For this review, take the finished solid that the model builds, in its own axes (mm). A direction names the side the tool comes from. Round coordinates to 2 decimals unless told otherwise and drop trailing zeros. Write each loop counter-clockwise with the first axis right and the second up, starting at its lowest first coordinate (ties: lowest second). Pieces come first, ordered by that corner, then holes.
from build123d import *

# Parameters (mm, degrees)
CROQUIS3_W               = 75.27
CROQUIS3_H               = 32.91
SALIENTE_EXTRUIR1_DEPTH  = 3.82
SALIENTE_EXTRUIR2_DEPTH  = 3.84
SALIENTE_EXTRUIR3_DEPTH  = 3.84
CROQUIS8_W               = 82.95
CROQUIS8_H               = 15.57
SALIENTE_EXTRUIR5_DEPTH  = 3.8
CROQUIS9_W               = 82.95
CROQUIS9_H               = 24.43
SALIENTE_EXTRUIR7_DEPTH  = 3.8
CROQUIS10_W              = 82.95
CROQUIS10_H              = 8.18
SALIENTE_EXTRUIR9_DEPTH  = 33.8
CROQUIS11_R              = 3.475
CORTAR_EXTRUIR3_DEPTH    = 33.8
SALIENTE_EXTRUIR10_DEPTH = 3.84
SALIENTE_EXTRUIR11_DEPTH = 3.84
CROQUIS15_R              = 3.9
SALIENTE_EXTRUIR12_DEPTH = 3.8


with BuildPart() as part:
    # Croquis3 → Saliente-Extruir1 (new body)
    with BuildSketch(Plane.XY):
        Rectangle(CROQUIS3_W, CROQUIS3_H)
    extrude(amount=SALIENTE_EXTRUIR1_DEPTH)

    # Croquis4 → Saliente-Extruir2 (add)
    with BuildSketch(Plane(origin=(37.635, 0, 0), x_dir=(0, 0, -1), z_dir=(1, 0, 0))):
        Polygon((-3.82, -16.455), (0, -16.455), (0, 16.455), (-3.82, 16.455), (-15.57, -16.455), align=None)
    extrude(amount=SALIENTE_EXTRUIR2_DEPTH)

    # Croquis5 → Saliente-Extruir3 (add)
    with BuildSketch(Plane.ZY.offset(37.635)):
        Polygon((3.82, -16.455), (0, -16.455), (0, 16.455), (3.82, 16.455), (15.57, -16.455), align=None)
    extrude(amount=SALIENTE_EXTRUIR3_DEPTH)

    # Croquis8 → Saliente-Extruir5 (add)
    with BuildSketch(Plane(origin=(0, -16.455, 0), x_dir=(-1, 0, 0), z_dir=(0, -1, 0))):
        with Locations((0, -7.785)):
            Rectangle(CROQUIS8_W, CROQUIS8_H)
    extrude(amount=SALIENTE_EXTRUIR5_DEPTH)

    # Croquis9 → Saliente-Extruir7 (add)
    with BuildSketch(Plane.XZ.offset(20.255)):
        with Locations((0, -12.215)):
            Rectangle(CROQUIS9_W, CROQUIS9_H)
    extrude(amount=-SALIENTE_EXTRUIR7_DEPTH)

    # Croquis10 → Saliente-Extruir9 (add)
    with BuildSketch(Plane(origin=(0, 16.455, 0), x_dir=(1, 0, 0), z_dir=(0, 1, 0))):
        with Locations((0, 4.09)):
            Rectangle(CROQUIS10_W, CROQUIS10_H)
    extrude(amount=-SALIENTE_EXTRUIR9_DEPTH)

    # Croquis11 → Cortar-Extruir3 (cut)
    with BuildSketch(Plane.XY.offset(3.82)):
        Circle(CROQUIS11_R)
    extrude(amount=-CORTAR_EXTRUIR3_DEPTH, mode=Mode.SUBTRACT)

    # Croquis12 → Saliente-Extruir10 (add)
    with BuildSketch(Plane(origin=(41.475, 0, 0), x_dir=(0, 0, -1), z_dir=(1, 0, 0))):
        Polygon((8.18, 16.455), (24.43, -16.455), (8.18, -16.455), align=None)
    extrude(amount=-SALIENTE_EXTRUIR10_DEPTH)

    # Croquis14 → Saliente-Extruir11 (add)
    with BuildSketch(Plane.ZY.offset(41.475)):
        Polygon((-8.18, 16.455), (-8.18, -16.772028127), (-24.43, -16.455), align=None)
    extrude(amount=-SALIENTE_EXTRUIR11_DEPTH)

    # Croquis15 → Saliente-Extruir12 (add)
    # profile 1 of 2: a face of its own
    with BuildSketch(Plane.XZ.offset(20.255)):
        with BuildLine():
            Line((41.475, 15.57), (41.475, -24.43))
            Line((41.475, -24.43), (52.99576157, -14.32670597))
            Line((52.99576157, -14.32670597), (52.99576157, -14.522664239))
            ThreePointArc((52.99576157, -14.522664239), (63.088425809, -4.43), (52.99576157, 5.662664239))
            Line((52.99576157, 5.662664239), (52.99576157, 5.858622508))
            Line((52.99576157, 5.858622508), (41.475, 15.57))
        make_face()
        with Locations(Location((52.99576157, -4.43, 0), (0, 0, 270))):
            Circle(CROQUIS15_R, mode=Mode.SUBTRACT)
    # profile 2 of 2: a face of its own
    with BuildSketch(Plane.XZ.offset(20.255)):
        with BuildLine():
            Line((-52.99576157, 5.858622508), (-41.475, 15.57))
            Line((-41.475, 15.57), (-41.475, -24.43))
            Line((-41.475, -24.43), (-52.99576157, -14.32670597))
            Line((-52.99576157, -14.32670597), (-52.99576157, -14.522664239))
            ThreePointArc((-52.99576157, -14.522664239), (-63.088425809, -4.43), (-52.99576157, 5.662664239))
            Line((-52.99576157, 5.662664239), (-52.99576157, 5.858622508))
        make_face()
        with Locations(Location((-52.99576157, -4.43, 0), (0, 0, 270))):
            Circle(CROQUIS15_R, mode=Mode.SUBTRACT)
    extrude(amount=-SALIENTE_EXTRUIR12_DEPTH)


solid = part.part
(1) For line 1 along X through (y, z) = (-18, -4); line 2 along Y through (x, z) = (0, -1.5) (3 decimals); line 3 along X through (y, z) = (0.5, -8.5) (3 decimals), list the stretches that pass through material, from the lowest coordinate up.
Geometry check:
line 1: x = -63.08 to -56.87, -49.12 to 49.12, 56.87 to 63.08
line 2: y = -20.255 to -3.475, 3.475 to 16.455
line 3: x = -41.475 to -37.635, 37.635 to 41.475
(2) We need section D-D, the plane x = 39. Give the boundary of the cut face in (y, z) (3 decimals).
Geometry check:
outline: (-20.255, -24.43) - (-16.455, -24.43) - (16.455, -8.18) - (16.455, 3.82) - (-16.455, 15.57) - (-20.255, 15.57) - close
(3) We need section B-B, the plane x = 0. Give the boundary of the cut face in (y, z) (3 decimals).
Geometry check:
outline: (-20.255, -24.43) - (-16.455, -24.43) - (-16.455, -8.18) - (-3.475, -8.18) - (-3.475, 3.82) - (-16.455, 3.82) - (-16.455, 15.57) - (-20.255, 15.57) - close; (3.475, -8.18) - (16.455, -8.18) - (16.455, 3.82) - (3.475, 3.82) - close
(4) For pin 1 Ø10 at (x, y) = (14, -5.5) entering from -Z; pin 2 Ø24 at (x, z) = (-57.5, -6) entering from +Y (3 decimals); pin 3 Ø6 at (y, z) = (9.5, 8) entering from +X (3 decimals); pin 4 Ø7 at (x, z) = (53, -4.43) entering from -Y, all flat-tipped, find the tip position at first contact; note any pin that passes through.
Geometry check:
pin 1: stops at z = -8.18
pin 2: stops at y = -16.455
pin 3: stops at x = 41.475
pin 4: passes through
(5) Mouldability with a two-part tool opening along X and no side actions: class faces 4 (the face through (-1, -18, -24.43)), 5 (the face through (41.475, -3, -5)), 6 (the face through (-63.086, -18.382, -4.652)), 7 (the face through (-1, 4, -8.18)) as pulls with the +X half, pulls with the -X half, needs draft (parallel to the pull), parting line crosses it, or undercut.
Geometry check:
face 4: needs draft
face 5: pulls with the +X half
face 6: pulls with the -X half
face 7: undercut
(6) We need section C-C, the plane y = 0. Give the boundary of the cut face in (x, z) (3 decimals), and give its area (3 significant figures).
Geometry check:
outline: (-41.475, -16.305) - (-37.635, -16.305) - (-37.635, -8.18) - (-3.475, -8.18) - (-3.475, 3.82) - (-37.635, 3.82) - (-37.635, 9.695) - (-41.475, 9.695) - close; (3.475, -8.18) - (37.635, -8.18) - (37.635, -16.305) - (41.475, -16.305) - (41.475, 9.695) - (37.635, 9.695) - (37.635, 3.82) - (3.475, 3.82) - close
area: 1,020 mm2
(7) We need section A-A, the plane z = -4.43. Give the boundary of the cut face in (x, y) (3 decimals).
Geometry check:
outline: (-63.088, -20.255) - (-56.896, -20.255) - (-56.896, -16.455) - (-63.088, -16.455) - close; (-49.096, -20.255) - (49.096, -20.255) - (49.096, -16.455) - (41.475, -16.455) - (41.475, 16.455) - (-41.475, 16.455) - (-41.475, -16.455) - (-49.096, -16.455) - close; (56.896, -20.255) - (63.088, -20.255) - (63.088, -16.455) - (56.896, -16.455) - close; hole circle Ø6.95 at (0, 0)
(8) For faces 1 (the face through (-1, -16.455, -16)), 2 (the face through (-39.58, -0.23, -16.42)), 3 (the face through (-1, 4, 3.82)), list the 3-axis set-ups (+Z, -Z, +X, -X, +Y, -Y) from which the entire face can be reached by the end or side of a thin tool; tool diameter is ignored.
Geometry check:
face 1: -Z, +Y
face 2: -Z, +X, -X, +Y
face 3: +Z, +Y
